Geometry check sheet. Reference: the model listing, model coordinates, mm. Face numbers are marked on the shaded views. A direction names the side the tool comes from. Round coordinates to 2 decimals unless told otherwise and drop trailing zeros. Write each loop counter-clockwise with the first axis right and the second up, starting at its lowest first coordinate (ties: lowest second). Pieces come first, ordered by that corner, then holes. Notation, with made-up numbers: (-35.5, 0) -> (1.5, 0) arc R31 ccw to (1.5, 26) -> close; hole circle Ø3 at (37, 77). An arc over 180 degrees is marked (long way). Use a Markdown table: item, result.
```python
from build123d import *

# Parameters (mm, degrees)
F0_R      = 40
F1_DEPTH  = 90
F2_R      = 25
F3_DEPTH  = 80
F4_R      = 17.5
F5_DEPTH  = 70
F7_DEPTH  = 30
F8_SIZE   = 1
F9_R      = 22.5
F10_DEPTH = 95
F11_SIZE  = 1


with BuildPart() as f1:
    # F0 (on Front) → F1 (new body)
    with BuildSketch(Plane.XZ):
        with Locations((40.362715, 0)):
            Circle(F0_R)
    extrude(amount=F1_DEPTH)

    # F2 (on face) → F3 (join)
    with BuildSketch(Plane.XZ.offset(90)):
        with Locations((40.362715, 0)):
            Circle(F2_R)
    extrude(amount=F3_DEPTH)

    # F4 (on face) → F5 (join)
    with BuildSketch(Plane.XZ.offset(170)):
        with Locations((40.362715, 0)):
            Circle(F4_R)
    extrude(amount=F5_DEPTH)

    # F6 (on Right) → F7 (cut)
    with BuildSketch(Plane.YZ):
        with BuildLine():
            ThreePointArc((-230, 5), (-235, 0), (-230, -5))
            Line((-230, -5), (-205, -5))
            ThreePointArc((-205, -5), (-200, 0), (-205, 5))
            Line((-205, 5), (-230, 5))
        make_face()
    extrude(amount=F7_DEPTH, mode=Mode.SUBTRACT)

    # F8
    f8_edges = [f1.edges().sort_by_distance(p)[0] for p in [
        (22.862715, -240, 0),
        (15.362715, -170, 0),
        (0.362715, -90, 0),
    ]]
    chamfer(f8_edges, length=F8_SIZE)

    # F9 (on face) → F10 (join)
    with BuildSketch(Plane(origin=(0, 0, 0), x_dir=(-1, 0, 0), z_dir=(0, 1, 0))):
        with Locations((-40.362715, 0)):
            Circle(F9_R)
    extrude(amount=F10_DEPTH)

    # F11
    f11_edges = [f1.edges().sort_by_distance(p)[0] for p in [
        (62.862715, 95, 0),
        (0.362715, 0, 0),
    ]]
    chamfer(f11_edges, length=F11_SIZE)


solid = f1.part
```
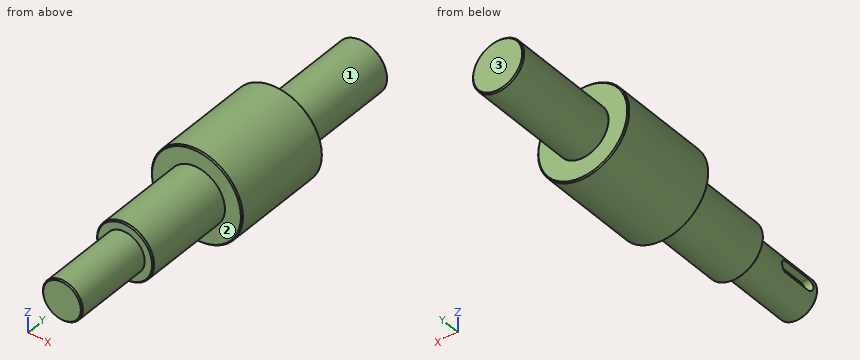
(1) Gauge pin test, flat ends, axial feed: pin 1 Ø7 at (x, y) = (26.5, -220) entering from +Z; pin 2 Ø8 at (y, z) = (-116.5, 19) entering from -X; pin 3 Ø12 at (y, z) = (-202, 16.5) entering from -X. Record the tip position at first contact, or that the pin passes through.
A:
| item | result |
|---|---|
| pin 1 | stops at z = 14.1 |
| pin 2 | stops at x = 20.36 |
| pin 3 | stops at x = 26.36 |
(2) Access from +Z, -Z, +X, -X, +Y, -Y to the whole of each face (thin tool, end or side, straight path). Record for the marked faces 1, 2 and 3.
A:
| item | result |
|---|---|
| face 1 | +Y |
| face 2 | -Y |
| face 3 | +Z, -Z, +X, -X, +Y |
(3) Section check B-B on y = -24. Record the cut outline in (x, z), plus the area to 3 significant figures.
A:
| item | result |
|---|---|
| outline | circle Ø80 at (40.36, 0) |
| area | 5,030 mm2 |
(4) Thickness scan on line 1 (Z direction, x = 41.5, y = -97.5); line 2 (Y direction, x = 57.5, z = -8); line 3 (Y direction, x = 18, z = 3). Record the ranges inside material, lowest first.
A:
| item | result |
|---|---|
| line 1 | z = -24.97 to 24.97 |
| line 2 | y = -170 to 95 |
| line 3 | y = -170 to 0 |
